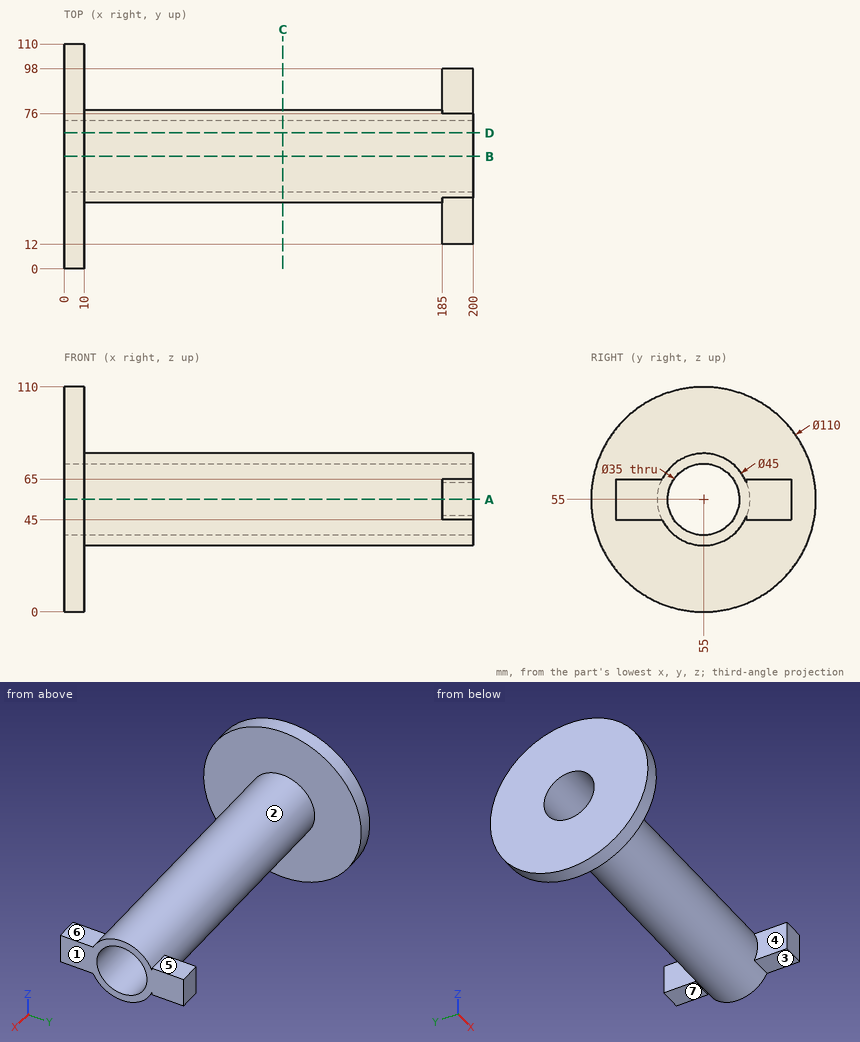
Here's the drawing with two shaded views (mm, measured from the low corner). I have some questions. A direction names the side the tool comes from. Coordinates: 2 decimals unless noted, no trailing zeros. Write each loop counter-clockwise with the first axis right and the second up, starting at its lowest first coordinate (ties: lowest second). Pieces come first, ordered by that corner, then holes.
Item 1: I want a section at C-C on x = 107. Write out the boundary of the cut face in (y, z).
Item 2: If we mould it in two halves opening along X, with no side actions, what happens to the marked faces 1, 2, 3 and 4? For each: +X half, -X half, draft (parallel to the pull), parting line (faces both ways), or undercut.
Item 3: I want a section at D-D on y = 66.5. Write out the boundary of the cut face in (x, z), and give its area (3 significant figures).
Item 4: I want a section at B-B on y = 55. Write out the boundary of the cut face in (x, z).
Item 5: If I drill on line 1 (Y direction, x = 66, z = 55); line 2 (X direction, y = 97, z = 27); line 3 (X direction, y = 14, z = 50), over which ranges is the centre line in solid material (lowest first)?
Item 6: Will these pins go through, and if not, where does the flat tip stop? pin 1 (16.5 mm diameter, centred on x = 196, y = 88, fed in from +Z); pin 2 (12 mm diameter, centred on x = 66, z = 56, fed in from -Y); pin 3 (5 mm diameter, centred on y = 85.5, z = 71, fed in from +X).
Item 7: I want a section at A-A on z = 55. Write out the boundary of the cut face in (x, y), and give its area (4 significant figures).
Item 8: On a 3-axis mill with a long thin cutter (end or side, diameter ignored), from which of +Z, -Z, +X, -X, +Y, -Y can I reach the whole of each face in a straight line? I mean the marked faces 5, 6 and 7. Say none if no direction works.
Findings below:
1. outline: circle Ø45 at (55, 55); hole circle Ø35 at (55, 55)
2. face 1: +X half
2. face 2: undercut
2. face 3: draft
2. face 4: undercut
3. outline: (0, 1.22) - (10, 1.22) - (10, 35.66) - (200, 35.66) - (200, 41.81) - (0, 41.81) - close; (0, 68.19) - (200, 68.19) - (200, 74.34) - (10, 74.34) - (10, 108.78) - (0, 108.78) - close
3. area: 3,150 mm2
4. outline: (0, 0) - (10, 0) - (10, 32.5) - (200, 32.5) - (200, 37.5) - (0, 37.5) - close; (0, 72.5) - (200, 72.5) - (200, 77.5) - (10, 77.5) - (10, 110) - (0, 110) - close
5. line 1: y = 32.5 to 37.5, 72.5 to 77.5
5. line 2: x = 0 to 10
5. line 3: x = 0 to 10, 185 to 200
6. pin 1: stops at z = 65
6. pin 2: stops at y = 32.5
6. pin 3: stops at x = 10
7. outline: (0, 0) - (10, 0) - (10, 32.5) - (185, 32.5) - (185, 12) - (200, 12) - (200, 37.5) - (0, 37.5) - close; (0, 72.5) - (200, 72.5) - (200, 98) - (185, 98) - (185, 77.5) - (10, 77.5) - (10, 110) - (0, 110) - close
7. area: 3,265 mm2
8. face 5: +Z, +X, +Y
8. face 6: +Z, +X, -Y
8. face 7: -Z, +X, +Y
